Could you check a few things on this model? Use its own coordinates, in mm. A direction names the side the tool comes from. Coordinates: 2 decimals unless noted, no trailing zeros. Order: outer loops, then holes, each group sorted by start corner. A loop starts at its lowest first (then second) coordinate and runs counter-clockwise, first axis right, second up. Notation, with made-up numbers: (-6, -31.5) - (23, -31.5) arc R13 ccw to (23, -11.5) - close; hole circle Ø2 at (38, 31.5). An arc over 180 degrees is marked (long way). Answer as a JSON object with one key per item and string values. Group by question number.
(1) Which directions (+Z, -Z, +X, -X, +Y, -Y) give clear straight access to the entire face, cutting with the end or side of a thin tool? Please do faces 5 (the cylindrical face through (0.715, -1.375, -0.493)), 6 (the flat face through (-0.1, -14.5, -5.6)), 7 (the flat face through (1, -3, -0.5)), 8 (the flat face through (0, -2, -1)), 9 (the flat face through (0, -9, -1)).
(2) Imagine slicing it at A-A, the plane x = 0. Write out the boundary of the cut face in (y, z) (3 decimals).
(3) Please list where these lines run through material, in increasing order: probe 1 along Y at (x, z) = (0, -0.2) (3 decimals); probe 2 along Y at (x, z) = (0, -0.75) (3 decimals); probe 3 along Z at (x, y) = (6.75, -8).
(4) Imagine slicing it at D-D, the plane z = -1.9. Write out the boundary of the cut face in (x, y), and give its area (3 significant figures).
(5) Imagine slicing it at C-C, the plane x = -9.5. Write out the boundary of the cut face in (y, z).
(6) Imagine slicing it at B-B, the plane y = 1.25. Write out the boundary of the cut face in (x, z), and give its area (3 significant figures).
(7) Will these pins go through, and if not, where does the flat tip stop? P1, Ø2.5, axis at x = 0.5, y = 0, coming from the -Z side; P2, Ø2, axis at y = -2, z = -1, coming from the +X side; P3, Ø4, axis at x = 0, y = 0, coming from the +Z side.
(8) We'd pull the mould along X, two halves only. Please class faces 1 (the cylindrical face through (-0.2, -15.1, -2.8)), 2 (the cylindrical face through (0.072, -3.474, -0.754)), 3 (the flat face through (6.609, -3.462, -0.493)), 4 (the cylindrical face through (-0.068, -2.974, -0.754)): pulls with the +X half, pulls with the -X half, needs draft (parallel to the pull), parting line crosses it, or undercut.
from build123d import *

# Parameters (mm, degrees)
CROQUIS1_R              = 1.55
SALIENTE_EXTRUIR1_DEPTH = 1
CROQUIS3_R              = 1.55
CORTAR_EXTRUIR1_DEPTH   = 0.5
SALIENTE_EXTRUIR2_DEPTH = 4.6


with BuildPart() as part:
    # Croquis1 → Saliente-Extruir1 (new body)
    with BuildSketch(Plane.XY):
        with BuildLine():
            Line((-1.573312588, 1.573312588), (-11.505819195, -8.359194019))
            ThreePointArc((-11.505819195, -8.359194019), (-11.797766675, -9.022819962), (-11.564578543, -9.709300857))
            ThreePointArc((-11.564578543, -9.709300857), (0, -15.1), (11.564578543, -9.709300857))
            ThreePointArc((11.564578543, -9.709300857), (11.797766675, -9.022819962), (11.505819195, -8.359194019))
            Line((11.505819195, -8.359194019), (1.573312588, 1.573312588))
            ThreePointArc((1.573312588, 1.573312588), (0, 2.225), (-1.573312588, 1.573312588))
        make_face()
        Circle(CROQUIS1_R, mode=Mode.SUBTRACT)
    extrude(amount=-SALIENTE_EXTRUIR1_DEPTH)

    # Croquis3 → Cortar-Extruir1 (cut)
    with BuildSketch(Plane(origin=(0, 0, -1), x_dir=(-1, 0, 0), z_dir=(0, 0, -1))):
        Circle(CROQUIS3_R)
        with BuildLine():
            Line((-2.969736593, 0.176888584), (-3.460771197, -0.314146021))
            ThreePointArc((-3.460771197, -0.314146021), (0, -3.475), (3.460771197, -0.314146021))
            Line((3.460771197, -0.314146021), (2.969736593, 0.176888584))
            ThreePointArc((2.969736593, 0.176888584), (0, -2.975), (-2.969736593, 0.176888584))
        make_face()
    extrude(amount=-CORTAR_EXTRUIR1_DEPTH, mode=Mode.SUBTRACT)

    # Croquis4 → Saliente-Extruir2 (add)
    with BuildSketch(Plane(origin=(0, 0, -1), x_dir=(-1, 0, 0), z_dir=(0, 0, -1))):
        with BuildLine():
            ThreePointArc((-11.559897122, -8.41776565), (0, -14.3), (11.559897122, -8.41776565))
            ThreePointArc((11.559897122, -8.41776565), (11.798705845, -9.062676129), (11.564578543, -9.709300857))
            ThreePointArc((11.564578543, -9.709300857), (0, -15.1), (-11.564578543, -9.709300857))
            ThreePointArc((-11.564578543, -9.709300857), (-11.798705845, -9.062676129), (-11.559897122, -8.41776565))
        make_face()
    extrude(amount=SALIENTE_EXTRUIR2_DEPTH)


solid = part.part
Result set:
{
 "1": {"face 5": "+Z, -Z", "face 6": "-Z, +X, -X, +Y, -Y", "face 7": "-Z", "face 8": "-Z, +X, -X, +Y", "face 9": "-Z, +Y"},
 "2": {"outline": "(-15.1, -5.6) - (-14.3, -5.6) - (-14.3, -1) - (-3.475, -1) - (-3.475, -0.5) - (-2.975, -0.5) - (-2.975, -1) - (-1.55, -1) - (-1.55, 0) - (-15.1, 0) - close; (1.55, -1) - (2.225, -1) - (2.225, 0) - (1.55, 0) - close"},
 "3": {"probe 1": "y = -15.1 to -1.55, 1.55 to 2.225", "probe 2": "y = -15.1 to -3.475, -2.975 to -1.55, 1.55 to 2.225", "probe 3": "z = -1 to 0"},
 "4": {"outline": "(-11.56, -9.71) arc R15.1 ccw to (11.56, -9.71) arc R1 ccw to (11.56, -8.42) arc R14.3 cw to (-11.56, -8.42) arc R1 ccw to start", "area": "21.7 mm^2"},
 "5": {"outline": "(-11.74, -5.6) - (-10.69, -5.6) - (-10.69, -1) - (-6.35, -1) - (-6.35, 0) - (-11.74, 0) - close"},
 "6": {"outline": "(-1.9, -1) - (-0.92, -1) - (-0.92, 0) - (-1.9, 0) - close; (0.92, -1) - (1.9, -1) - (1.9, 0) - (0.92, 0) - close", "area": "1.96 mm^2"},
 "7": {"P1": "stops at z = -1", "P2": "stops at x = 6.15", "P3": "stops at z = 0"},
 "8": {"face 1": "parting line crosses it", "face 2": "undercut", "face 3": "pulls with the +X half", "face 4": "undercut"}
}
